Source: CAD feature listing. Evaluate the final solid. Frame: model axes, mm. A direction names the side the tool comes from. Give positions to 0.01 mm unless a question says otherwise; leave off trailing zeros. Order: outer loops, then holes, each group sorted by start corner. A loop starts at its lowest first (then second) coordinate and runs counter-clockwise, first axis right, second up. Notation, with made-up numbers: M 48,-28.5 L 87,-28.5 A7 ccw 87,-19.5 Z; hole C 22.5,84 d6. An arc over 180 degrees is marked long. Answer in a Markdown table with one row per item. Add a question column.
(1) Section query A-A, the plane y = 175. Return loops of the section in (x, z).
(2) Section query B-B, the plane y = 50. Return loops of the section in (x, z), plus the area to 3 significant figures.
(3) Set-up query: faces 1 (the face through (0, 0, 0)), 2 (the face through (-9.837, 96.514, -0.028)). Return all of +Z, -Z, +X, -X, +Y, -Y with unobstructed straight access to the full face (end or side cutting, diameter ignored); none if empty.
(4) Section query C-C, the plane z = 0.8. Count the separate pieces of the cut face and the enclosed holes in it, plus the area to 3 significant figures.
(5) Mould query, pull axis Y, two halves, no side actions, for faces 3 (the face through (0, 161.539, 0)), 4 (the face through (17.885, 233.511, -0.028)), 5 (the face through (0, 21, 0)), 6 (the face through (-17.71, 75.08, -0.03)). Classes: pulls with the +Y half, pulls with the -Y half, needs draft (parallel to the pull), parting line crosses it, or undercut.
(6) Material intervals for line 1 along X through (y, z) = (200, -0.95); line 2 along X through (y, z) = (207, -0.05); line 3 along X through (y, z) = (79, 1.1), sorted ascending.
(7) Pin query (flat end, axial travel): P1, Ø1.5, axis at x = 3, y = 79, coming from the +Z side; P2, Ø2, axis at y = 109.5, z = 0.5, coming from the -X side; P3, Ø2, axis at x = 12, z = 0.5, coming from the -Y side. Return the tip coordinate at first contact, or that it passes through.
Autodesk Inventor part; units mm, degrees
ref_plane "YZ Plane" through (0, 0, 0) normal (1, 0, 0) x (0, 1, 0)
ref_plane "XZ Plane" through (0, 0, 0) normal (0, 1, 0) x (-1, 0, 0)
ref_plane "XY Plane" through (0, 0, 0) normal (0, 0, 1) x (1, 0, 0)
sketch "Sketch1" plane through (0, 0, 0) normal (0, 0, 1) x (1, 0, 0)
  line L0 (0, 0) -> (-7, 0)
  line L1 (-7, 0) -> (-11.5963, 3.8567)
  line L2 (-11.5963, 3.8567) -> (-24, 148.3252)
  line L3 (-24, 148.3252) -> (-24, 216.3252)
  line L4 (-24, 216.3252) -> (-11.5963, 251.1842)
  line L5 (-11.5963, 251.1842) -> (-7, 255.0409)
  line L6 (-7, 255.0409) -> (0, 255.0409)
  line L7 (0, 255.0409) -> (0, 0)
  line L8 (0, 6) -> (-4, 6)
  line L9 (-4, 6) -> (-4, 21)
  line L10 (-4, 21) -> (0, 21)
  line L11 (-5.5, 46) -> (-2.5, 46)
  line L12 (-2.5, 46) -> (-2.5, 125.6208)
  line L13 (-2.5, 125.6208) -> (-14.0543, 145.6334)
  line L14 (-14.0543, 145.6334) -> (-5.5, 46)
  line L15 (0, 249.0409) -> (-5, 249.0409)
  line L16 (-5, 249.0409) -> (-7.135, 243.0409)
  line L17 (-7.135, 243.0409) -> (0, 238.9899)
  line L18 (-8.7779, 238.224) -> (-2.5, 234.6596)
  line L19 (-2.5, 234.6596) -> (-2.5, 220.224)
  line L20 (-2.5, 220.224) -> (-15.1828, 220.224)
  line L21 (-15.1828, 220.224) -> (-8.7779, 238.224)
  line L22 (0, 131.2907) -> (-14, 155.5394)
  line L23 (-14, 155.5394) -> (0, 155.5394)
  arc A0 (0, 204) -> (0, 196) centre (0, 200) ccw
  circle A1 centre (-7, 200) radius 1.5
  line L24 (0, 0) -> (7, 0)
  line L25 (7, 0) -> (11.5963, 3.8567)
  line L26 (11.5963, 3.8567) -> (24, 148.3252)
  line L27 (24, 148.3252) -> (24, 216.3252)
  line L28 (24, 216.3252) -> (11.5963, 251.1842)
  line L29 (11.5963, 251.1842) -> (7, 255.0409)
  line L30 (7, 255.0409) -> (0, 255.0409)
  line L31 (0, 6) -> (4, 6)
  line L32 (4, 6) -> (4, 21)
  line L33 (4, 21) -> (0, 21)
  line L34 (5.5, 46) -> (2.5, 46)
  line L35 (2.5, 46) -> (2.5, 125.6208)
  line L36 (2.5, 125.6208) -> (14.0543, 145.6334)
  line L37 (14.0543, 145.6334) -> (5.5, 46)
  line L38 (0, 249.0409) -> (5, 249.0409)
  line L39 (5, 249.0409) -> (7.135, 243.0409)
  line L40 (7.135, 243.0409) -> (0, 238.9899)
  line L41 (8.7779, 238.224) -> (2.5, 234.6596)
  line L42 (2.5, 234.6596) -> (2.5, 220.224)
  line L43 (2.5, 220.224) -> (15.1828, 220.224)
  line L44 (15.1828, 220.224) -> (8.7779, 238.224)
  line L45 (0, 131.2907) -> (14, 155.5394)
  line L46 (14, 155.5394) -> (0, 155.5394)
  arc A2 (0, 196) -> (0, 204) centre (0, 200) ccw
  circle A3 centre (-16.5993, 116.8252) radius 2
  circle A4 centre (16.5993, 116.8252) radius 2
  circle A5 centre (-8.5, 27) radius 2
  circle A6 centre (8.5, 27) radius 2
  line L47 (0, 200) -> (-10, 200)
  line L48 (0, 204) -> (-14, 204)
  line L49 (0, 196) -> (-14, 196)
  circle A7 centre (-4.9497, 195.0503) radius 1.5
  circle A8 centre (0, 193) radius 1.5
  circle A9 centre (4.9497, 195.0503) radius 1.5
  circle A10 centre (7, 200) radius 1.5
  circle A11 centre (0, 207) radius 1.5
  line L50 (-24, 158.5394) -> (24, 158.5394)
  line L51 (0, 185.7881) -> (-14, 161.5394)
  line L52 (-14, 161.5394) -> (0, 161.5394)
  line L53 (14, 161.5394) -> (0, 161.5394)
  line L54 (0, 185.7881) -> (14, 161.5394)
  dimension "d0" = 7
  dimension "d1" = 6
  dimension "d2" = 145
  dimension "d3" = 68
  dimension "d4" = 37
  dimension "d5" = 48
  dimension "d8" = 140
  dimension "d9" = 140
  dimension "d10" = 15
  dimension "d11" = 6
  dimension "d12" = 4
  dimension "d13" = 3
  dimension "d14" = 5
  dimension "d15" = 25
  dimension "d17" = 100
  dimension "d19" = 5
  dimension "d20" = 28
  dimension "d21" = 150
  dimension "d29" = 6
  dimension "d32" = 6
  dimension "d33" = 4
  dimension "d38" = 3
  dimension "d42" = 4
  dimension "d43" = 31.5
  dimension "d45" = 5
  dimension "d46" = 4
  dimension "d47" = 17
  dimension "d48" = 6
  dimension "d51" = 200
  dimension "d54" = 3
  dimension "d56" = 14
  dimension "d57" = 8
  dimension "d58" = 7
  dimension "d61" = 180
  dimension "d63" = 5
  dimension "d64" = 5
  dimension "d65" = 100
  dimension "d66" = 7
  dimension "d67" = 5
  dimension "d68" = 18
  dimension "d69" = 6
extrude "Extrusion1" add sketch "Sketch1" along normal mid plane 4 contours L0 L1 L2 L3 L50 L7 L23 L22 L10 L9 L8 | L7 L31 L32 L33 L45 L46 L50 L27 L26 L25 L24 | L3 L4 L5 L6 L7 L15 L16 L17 A11 A0 A8 L51 L52 L50 | L50 L7 L53 L54 A8 A2 A11 L40 L39 L38 L30 L29 L28 L27 | L52 L51 L7 | L7 L54 L53 | A8 L7 | L7 A8 | A11 L7 | L7 A11
extrude "Extrusion2" cut sketch "Sketch1" along normal mid plane 10 contours L52 L51 L7 | L7 L54 L53 | A8 L7 | L7 A8 | A11 L7 | L7 A11
properties part number "Leg_part3"
Values follow:
| question | item | result |
|---|---|---|
| 1 | outline | M -24,-2 L -6.23,-2 L -6.23,2 L -24,2 Z; M 6.23,-2 L 24,-2 L 24,2 L 6.23,2 Z |
| 2 | outline | M -15.56,-2 L -5.84,-2 L -5.84,2 L -15.56,2 Z; M -2.5,-2 L 2.5,-2 L 2.5,2 L -2.5,2 Z; M 5.84,-2 L 15.56,-2 L 15.56,2 L 5.84,2 Z |
| 2 | area | 97.7 mm² |
| 3 | face 1 | +Z, -Z, +X, -X, -Y |
| 3 | face 2 | +Z, -Z |
| 4 | separate pieces | 1 |
| 4 | enclosed holes | 19 |
| 4 | area | 7,210 mm² |
| 5 | face 3 | undercut |
| 5 | face 4 | pulls with the +Y half |
| 5 | face 5 | undercut |
| 5 | face 6 | pulls with the -Y half |
| 6 | line 1 | x = -24 to -8.5, -5.5 to -4, 4 to 5.5, 8.5 to 24 |
| 6 | line 2 | x = -24 to -1.5, 1.5 to 24 |
| 6 | line 3 | x = -18.05 to -8.33, -2.5 to 2.5, 8.33 to 18.05 |
| 7 | P1 | stops at z = 2 |
| 7 | P2 | stops at x = -20.75 |
| 7 | P3 | stops at y = 3.36 |
